```python
from build123d import *
from build123d.topology import SkipClean

# Parameters (mm, degrees)
SKETCH2_R           = 7.5
BOSS_EXTRUDE1_DEPTH = 10
FILLET1_R           = 5
BOSS_EXTRUDE2_START = -24
SKETCH3_R           = 11
SKETCH3_R_2         = 7.5
BOSS_EXTRUDE2_DEPTH = 24
CUT_EXTRUDE1_REACH  = 135.566
SKETCH4_R           = 1.55
SKETCH6_W           = 37.11251069
SKETCH6_H           = 1
CUT_EXTRUDE3_DEPTH  = 10
SKETCH7_W           = 36.737317401
SKETCH7_H           = 1
CUT_EXTRUDE4_DEPTH  = 3
FILLET2_R           = 5
SKETCH8_R           = 1.5
CUT_EXTRUDE5_DEPTH  = 7
SKETCH9_W           = 1.241983996
SKETCH9_H           = 1.188202975
CUT_EXTRUDE6_DEPTH  = 1


with BuildPart() as part:
    # Sketch2 → Boss-Extrude1 (new body)
    with BuildSketch(Plane.XY):
        with BuildLine():
            Line((-22.5, 3.831552556), (-22.5, 14.831552556))
            Line((-22.5, 14.831552556), (-12.5, 14.831552556))
            Line((-12.5, 14.831552556), (-12.5, 3.831552556))
            Line((-12.5, 3.831552556), (-2.5, 3.831552556))
            Line((-2.5, 3.831552556), (-2.5, 14.831552556))
            Line((-2.5, 14.831552556), (7.5, 14.831552556))
            Line((7.5, 14.831552556), (7.5, 3.831552556))
            Line((7.5, 3.831552556), (88.192235936, 3.831552556))
            ThreePointArc((88.192235936, 3.831552556), (91.819805392, 9.932478429), (98.5, 12.331552556))
            ThreePointArc((98.5, 12.331552556), (109, 1.831552556), (98.5, -8.668447444))
            Line((98.5, -8.668447444), (-98.5, -8.668447444))
            ThreePointArc((-98.5, -8.668447444), (-109, 1.831552556), (-98.5, 12.331552556))
            ThreePointArc((-98.5, 12.331552556), (-91.358571571, 9.975203317), (-87.021759717, 3.831552556))
            Line((-87.021759717, 3.831552556), (-22.5, 3.831552556))
        make_face()
        with Locations((-98.5, 1.831552556)):
            Circle(SKETCH2_R, mode=Mode.SUBTRACT)
        with Locations((98.5, 1.831552556)):
            Circle(SKETCH2_R, mode=Mode.SUBTRACT)
    extrude(amount=BOSS_EXTRUDE1_DEPTH)

    # Fillet1
    fillet1_edges = [part.edges().sort_by_distance(p)[0] for p in [
        (88.192235936, 3.831552556, 5),
    ]]
    fillet(fillet1_edges, radius=FILLET1_R)

    # Sketch3 → Boss-Extrude2 (add)
    with BuildSketch(Plane.XY.offset(10).offset(BOSS_EXTRUDE2_START)):
        with Locations((-98.5, 1.831552556)):
            Circle(SKETCH3_R)
        with Locations((-98.5, 1.831552556)):
            Circle(SKETCH3_R_2, mode=Mode.SUBTRACT)
    boss_extrude2 = extrude(amount=BOSS_EXTRUDE2_DEPTH)

    # Mirror1: Boss-Extrude2 across plane
    with SkipClean():  # the faces are left unmerged after this step: merging them gives an invalid solid
        add(boss_extrude2.mirror(Plane(origin=(0, 0, 0), x_dir=(0, 0, 1), z_dir=(1, 0, 0))))

    # Cut-Extrude1: up to this face of the body (flat: up to its plane)
    cut_extrude1_end = Plane(part.part.faces().sort_by_distance((7.5, 9.331552556, 5))[0])
    # Sketch4 → Cut-Extrude1 (cut, up to the picked face)
    with BuildSketch(Plane.ZY.offset(22.5), mode=Mode.PRIVATE) as cut_extrude1_sk1:
        with Locations((5, 10.805752832)):
            Circle(SKETCH4_R)
    cut_extrude1_tool1 = split(extrude(cut_extrude1_sk1.sketch, amount=-CUT_EXTRUDE1_REACH, mode=Mode.PRIVATE), bisect_by=cut_extrude1_end, keep=Keep.BOTH, mode=Mode.PRIVATE)
    add(cut_extrude1_tool1.solids().sort_by(Axis((-22.5, 10.805753, 5), (1, 0, 0)))[0], mode=Mode.SUBTRACT)

    # Sketch6 → Cut-Extrude3 (cut)
    with BuildSketch(Plane(origin=(110, 0, 0), x_dir=(0, 0, -1), z_dir=(1, 0, 0))):
        with Locations((1.381927251, 1.831552556)):
            Rectangle(SKETCH6_W, SKETCH6_H)
    cut_extrude3 = extrude(amount=-CUT_EXTRUDE3_DEPTH, mode=Mode.SUBTRACT)

    # Mirror2: Cut-Extrude3 across plane
    add(cut_extrude3.mirror(Plane(origin=(0, 0, 0), x_dir=(0, 0, 1), z_dir=(1, 0, 0))), mode=Mode.SUBTRACT)

    # Sketch7 → Cut-Extrude4 (cut)
    with BuildSketch(Plane(origin=(0, 14.831552556, 0), x_dir=(1, 0, 0), z_dir=(0, 1, 0))):
        with Locations((-7.879171978, -4.654369626)):
            Rectangle(SKETCH7_W, SKETCH7_H)
    extrude(amount=-CUT_EXTRUDE4_DEPTH, mode=Mode.SUBTRACT)

    # Fillet2
    fillet2_edges = [part.edges().sort_by_distance(p)[0] for p in [
        (-87.021759717, 3.831552556, 5),
    ]]
    fillet(fillet2_edges, radius=FILLET2_R)

    # Sketch8 → Cut-Extrude5 (cut)
    with BuildSketch(Plane(origin=(0, 3.831552556, 0), x_dir=(1, 0, 0), z_dir=(0, 1, 0))):
        with Locations(Location((-66.25676189, -5, 0), (0, 0, 270))):
            Circle(SKETCH8_R)
        with Locations(Location((-54.25676189, -5, 0), (0, 0, 270))):
            Circle(SKETCH8_R)
        with Locations(Location((-32.502764064, -5, 0), (0, 0, 270))):
            Circle(SKETCH8_R)
        with Locations(Location((32.497235936, -5, 0), (0, 0, 270))):
            Circle(SKETCH8_R)
        with Locations(Location((54.24523811, -5, 0), (0, 0, 270))):
            Circle(SKETCH8_R)
        with Locations(Location((66.24523811, -5, 0), (0, 0, 270))):
            Circle(SKETCH8_R)
    extrude(amount=-CUT_EXTRUDE5_DEPTH, mode=Mode.SUBTRACT)

    # Sketch9 → Cut-Extrude6 (cut)
    with BuildSketch(Plane(origin=(0, 3.831552556, 0), x_dir=(1, 0, 0), z_dir=(0, 1, 0))):
        with Locations((-80.613746542, -5.894733375)):
            Rectangle(SKETCH9_W, SKETCH9_H)
    extrude(amount=-CUT_EXTRUDE6_DEPTH, mode=Mode.SUBTRACT)


solid = part.part
```
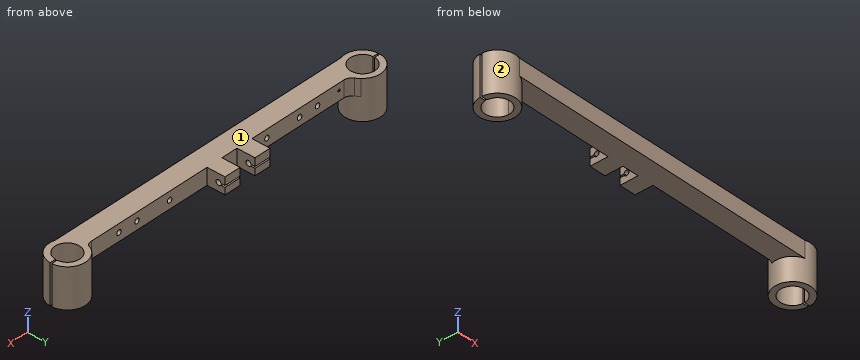
The listing builds one solid part. Answer for the finished solid, in the listing's coordinates (mm). Face numbers are marked on the shaded views. Give positions to 0.01 mm unless a question says otherwise; leave off trailing zeros. Order: outer loops, then holes, each group sorted by start corner. A loop starts at its lowest first (then second) coordinate and runs counter-clockwise, first axis right, second up. Notation, with made-up numbers: (7, 67.5) -> (32, 67.5) arc R21 cw to (32, 102.5) -> close; hole circle Ø3 at (32, 62). An arc over 180 degrees is marked (long way). Answer as a JSON object with one key per item and string values. Group by question number.
Item 1: Determine the mould class of the marked faces 1 and 2 for opening direction X: pulls with the +X half, pulls with the -X half, needs draft (parallel to the pull), parting line crosses it, or undercut.
Item 2: The part is cut by section B-B on z = -4. Write down the section's boundary in (x, y).
Item 3: The part is cut by section A-A on x = 98.5. Write down the section's boundary in (y, z).
Item 4: The part is cut by section C-C on x = -29. Write down the section's boundary in (y, z).
Item 5: Consider L1, parallel to Z at x = 27, y = -5.25; L2, parallel to X at y = 9.5, z = -5; L3, parallel to X at y = 0.5, z = 3.25. Determine where each line is inside the solid, lowest interval first. Write a range as from..to.
Item 6: Flat-ended cylindrical pins translate along their axes: pin 1 (12 mm diameter, centred on x = 31.5, z = 0, fed in from -Y); pin 2 (12 mm diameter, centred on x = -78.5, y = 8, fed in from -Z); pin 3 (3 mm diameter, centred on y = 6, z = 4, fed in from -X). Find the tip coordinate at first contact, or state that the pin passes through.
Result set:
{
 "1": {"face 1": "needs draft", "face 2": "undercut"},
 "2": {"outline": "(-109.49, 1.33) arc R11 ccw (long way) to (-109.49, 2.33) -> (-105.98, 2.33) arc R7.5 cw (long way) to (-105.98, 1.33) -> close; (105.98, 1.33) arc R7.5 cw (long way) to (105.98, 2.33) -> (109.49, 2.33) arc R11 ccw (long way) to (109.49, 1.33) -> close"},
 "3": {"outline": "(-9.17, -14) -> (-5.67, -14) -> (-5.67, 10) -> (-9.17, 10) -> close; (9.33, -14) -> (12.83, -14) -> (12.83, 10) -> (9.33, 10) -> close"},
 "4": {"outline": "(-8.67, 0) -> (3.83, 0) -> (3.83, 10) -> (-8.67, 10) -> close"},
 "5": {"L1": "0..10", "L2": "-106.39..-90.61, 90.61..106.39", "L3": "-109.42..-105.88, -91.12..91.12, 105.88..109.42"},
 "6": {"pin 1": "y = -8.67", "pin 2": "z = 0", "pin 3": "x = -109.17"}
}
